Geometry check sheet. Reference: the model listing, model coordinates, mm. A direction names the side the tool comes from. Round coordinates to 2 decimals unless told otherwise and drop trailing zeros. Order: outer loops, then holes, each group sorted by start corner. A loop starts at its lowest first (then second) coordinate and runs counter-clockwise, first axis right, second up.
(1) Cross-section at A-A on z = 0.55. Enter the section's corners in (x, y).
(2) Draft check along X on faces 4 (the face through (0, 3, 4.8)), 5 (the face through (-2.422, 2.422, 4.52)), 6 (the face through (-0.9, 6.84, 2.37)). Enter one of: pulls with the +X half, pulls with the -X half, needs draft (parallel to the pull), parting line crosses it, or undercut.
(3) Gauge pin test, flat ends, axial feed: P1, Ø2, axis at x = -0.5, z = 3, coming from the +Y side; P2, Ø2, axis at x = 4.5, y = 2, coming from the -Z side. Record the tip position at first contact, or that the pin passes through.
(4) Thickness scan on L1, parallel to Y at x = 0, z = 1.05; L2, parallel to Z at x = 1.25, y = 5; L3, parallel to X at y = -1.25, z = 2.2. Record the ranges inside material, lowest first.
(5) Set-up check for faces 1 (the face through (-2.422, 2.422, 0.28)), 2 (the face through (0, 6, 4.681)), 3 (the face through (-0.338, 2.578, 2.366)): record each of +Z, -Z, +X, -X, +Y, -Y from which the full face is reachable in a straight line by a thin tool's end or side.
(6) Cross-section at B-B on z = 2.2. Enter the section's corners in (x, y), and give its area (3 significant figures).
from build123d import *

# Parameters (mm, degrees)
SKETCH1_R           = 6.9
SKETCH1_R_2         = 2.6
BOSS_EXTRUDE1_DEPTH = 4.8


with BuildPart() as part:
    # Sketch1 → Boss-Extrude1 (new body)
    with BuildSketch(Plane.XY):
        Circle(SKETCH1_R)
        Circle(SKETCH1_R_2, mode=Mode.SUBTRACT)
    extrude(amount=BOSS_EXTRUDE1_DEPTH)

    # Sketch2 → Cut-Revolve1 (revolve, cut)
    with BuildSketch(Plane(origin=(0, 0, 0), x_dir=(0, 0, -1), z_dir=(1, 0, 0)), mode=Mode.PRIVATE) as cut_revolve1_sk:
        Polygon((-5.047973747, 6.3), (-4.9457756, 6.3), (-4.9457756, 6.684089002), (-4.6811872, 6.419500602), (-4.6811872, 5.658380737), (-4.519629847, 5.81993809), (-4.422921243, 5.723229486), (-4.519629847, 5.626520881), (-4.519629847, 3.272939667), (-3.81743033, 3.272939667), (-3.81743033, 3.2), (-4.879732163, 3.2), (-4.879732163, 0), (-5.869193326, 0), (-5.869193326, 6.3), align=None)
        Polygon((1.069193326, 6.3), (0.247973747, 6.3), (0.1457756, 6.3), (0.1457756, 6.684089002), (-0.1188128, 6.419500602), (-0.1188128, 5.658380737), (-0.280370153, 5.81993809), (-0.377078757, 5.723229486), (-0.280370153, 5.626520881), (-0.280370153, 3.272939667), (-0.98256967, 3.272939667), (-0.98256967, 3.2), (0.079732163, 3.2), (0.079732163, 0), (1.069193326, 0), align=None)
    revolve(cut_revolve1_sk.sketch.rotate(Axis((0, 0, 4.879732163), (0, 0, 1)), 90), axis=Axis((0, 0, 4.879732163), (0, 0, 1)), mode=Mode.SUBTRACT)


solid = part.part
Found:
1. outline: circle Ø13.8 at (0, 0); circle Ø6.4 at (0, 0); hole circle Ø6.55 at (0, 0); hole circle Ø5.2 at (0, 0)
2. face 4: needs draft
2. face 5: undercut
2. face 6: parting line crosses it
3. P1: stops at y = 6.9
3. P2: stops at z = 0.12
4. L1: y = -6.9 to -2.6, 2.6 to 6.9
4. L2: z = 0.28 to 4.52
4. L3: x = -6.79 to -2.28, 2.28 to 6.79
5. face 1: -Z
5. face 2: +Z
5. face 3: +Z, -Z
6. outline: circle Ø13.8 at (0, 0); hole circle Ø5.2 at (0, 0)
6. area: 128 mm2
